The model under review builds one solid part; all positions refer to its coordinate system, in mm. A direction names the side the tool comes from. Give positions to 0.01 mm unless a question says otherwise; leave off trailing zeros. Order: outer loops, then holes, each group sorted by start corner. A loop starts at its lowest first (then second) coordinate and runs counter-clockwise, first axis right, second up. Notation, with made-up numbers: (12.5, 64.25) - (67.5, 64.25) arc R31 ccw to (67.5, 91.25) - close; hole circle Ø10 at (-15, 33.25). An arc over 180 degrees is marked (long way). Answer as CSV lines item,"result". Start each with the question number.
from build123d import *

# Parameters (mm, degrees)
F0_R     = 5
F0_W     = 3
F0_H     = 15
F0_R_2   = 3
F1_DEPTH = 3
F0_H_2   = 30
F2_DEPTH = 8
F3_DEPTH = 6
F4_DEPTH = 5


with BuildPart() as f1:
    # F0 (on Top) → F1 (new body)
    with BuildSketch(Plane.XY):
        Polygon((52, 30), (0, 30), (0, 0), (52, 0), (52, 7.5), (52, 22.5), align=None)
        with Locations((47, 7.5)):
            Circle(F0_R, mode=Mode.SUBTRACT)
        with Locations((11, 15)):
            Rectangle(F0_W, F0_H, mode=Mode.SUBTRACT)
        with Locations((23.5, 15)):
            Rectangle(F0_W, F0_H, mode=Mode.SUBTRACT)
        with Locations((36, 15)):
            Rectangle(F0_W, F0_H, mode=Mode.SUBTRACT)
        with Locations((47, 22.5)):
            Circle(F0_R, mode=Mode.SUBTRACT)
        with Locations((47, 7.5)):
            Circle(F0_R)
        with Locations((47, 7.5)):
            Circle(F0_R_2, mode=Mode.SUBTRACT)
        with Locations((47, 22.5)):
            Circle(F0_R)
        with Locations((47, 22.5)):
            Circle(F0_R_2, mode=Mode.SUBTRACT)
    extrude(amount=F1_DEPTH)

    # F0 (on Top) → F2 (join, through all)
    with BuildSketch(Plane.XY):
        with Locations((-1.5, 15)):
            Rectangle(F0_W, F0_H_2)
    extrude(amount=F2_DEPTH)

    # F0 (on Top) → F3 (join, through all)
    with BuildSketch(Plane.XY):
        with Locations((11, 15)):
            Rectangle(F0_W, F0_H)
        with Locations((23.5, 15)):
            Rectangle(F0_W, F0_H)
        with Locations((36, 15)):
            Rectangle(F0_W, F0_H)
    extrude(amount=F3_DEPTH)

    # F0 (on Top) → F4 (join, through all)
    with BuildSketch(Plane.XY):
        with Locations((47, 22.5)):
            Circle(F0_R)
        with Locations((47, 22.5)):
            Circle(F0_R_2, mode=Mode.SUBTRACT)
        with Locations((47, 7.5)):
            Circle(F0_R)
        with Locations((47, 7.5)):
            Circle(F0_R_2, mode=Mode.SUBTRACT)
    extrude(amount=F4_DEPTH)


solid = f1.part
Item 1: Machinability: for faces 4 (the face through (22, 15, 4)), 5 (the face through (36, 7.5, 4)), 6 (the face through (20, 15, 3)), 7 (the face through (23, 15, 6)), 8 (the face through (11, 22.5, 4)), which of the approach directions +Z, -Z, +X, -X, +Y, -Y give a long, thin tool a straight path to every point of the face, cutting with its end or side? Answer none if there is none.
Item 2: Mouldability with a two-part tool opening along Y and no side actions: class faces 1 (the face through (44, 22.6, 2.5)), 2 (the face through (23, 22.5, 4)), 3 (the face through (-2, 15, 8)) as released by +Y, released by -Y, zero draft, split by the parting line, or undercut.
Item 3: Take a section at B-B on z = 4. Write out the cut boundary in (x, y), and give its area (3 significant figures).
Item 4: Take a section at D-D on z = 1.25. Write out the cut boundary in (x, y).
Item 5: For line 1 along Y through (x, z) = (47, 1.65); line 2 along X through (y, z) = (13, 3.25); line 3 along X through (y, z) = (7, 7), list the stretches that pass through material, from the lowest coordinate up.
Item 6: Clearance check with flat-ended pins moving along their axes: pin 1 (1 mm diameter, centred on x = 20.5, y = 11, fed in from +Z); pin 2 (9.5 mm diameter, centred on x = 47, y = 7.5, fed in from +Z); pin 3 (5 mm diameter, centred on x = 47, y = 22.5, fed in from +Z); pin 4 (4 mm diameter, centred on x = 13.5, y = 7.5, fed in from +Z). State where each tip first meets the part, or that it passes through.
Item 7: Take a section at A-A on x = 47. Write out the cut boundary in (y, z).
Item 8: Take a section at C-C on y = 5.75. Write out the cut boundary in (x, z), and give its area (3 significant figures).
Data:
1,face 4,"+Z, +Y, -Y"
1,face 5,"+Z, -Y"
1,face 6,"+Z"
1,face 7,"+Z, +X, +Y, -Y"
1,face 8,"+Z, +Y"
2,face 1,"undercut"
2,face 2,"released by +Y"
2,face 3,"zero draft"
3,outline,"(-3, 0) - (0, 0) - (0, 30) - (-3, 30) - close; (9.5, 7.5) - (12.5, 7.5) - (12.5, 22.5) - (9.5, 22.5) - close; (22, 7.5) - (25, 7.5) - (25, 22.5) - (22, 22.5) - close; (34.5, 7.5) - (37.5, 7.5) - (37.5, 22.5) - (34.5, 22.5) - close; circle Ø10 at (47, 7.5); circle Ø10 at (47, 22.5); hole circle Ø6 at (47, 7.5); hole circle Ø6 at (47, 22.5)"
3,area,"326 mm^2"
4,outline,"(-3, 0) - (52, 0) - (52, 30) - (-3, 30) - close; hole circle Ø6 at (47, 7.5); hole circle Ø6 at (47, 22.5)"
5,line 1,"y = 0 to 4.5, 10.5 to 19.5, 25.5 to 30"
5,line 2,"x = -3 to 0, 9.5 to 12.5, 22 to 25, 34.5 to 37.5"
5,line 3,"x = -3 to 0"
6,pin 1,"stops at z = 3"
6,pin 2,"stops at z = 5"
6,pin 3,"passes through"
6,pin 4,"stops at z = 6"
7,outline,"(0, 0) - (4.5, 0) - (4.5, 5) - (2.5, 5) - (2.5, 3) - (0, 3) - close; (10.5, 0) - (19.5, 0) - (19.5, 5) - (17.5, 5) - (17.5, 3) - (12.5, 3) - (12.5, 5) - (10.5, 5) - close; (25.5, 0) - (30, 0) - (30, 3) - (27.5, 3) - (27.5, 5) - (25.5, 5) - close"
8,outline,"(-3, 0) - (44.56, 0) - (44.56, 5) - (42.32, 5) - (42.32, 3) - (0, 3) - (0, 8) - (-3, 8) - close; (49.44, 0) - (52, 0) - (52, 3) - (51.68, 3) - (51.68, 5) - (49.44, 5) - close"
8,area,"174 mm^2"
